from build123d import *

# Parameters (mm, degrees)
CYLINDER040_R     = 3.25
CYLINDER040_DEPTH = 2
CYLINDER041_R     = 3.25
CYLINDER041_DEPTH = 2
CYLINDER042_R     = 3.25
CYLINDER042_DEPTH = 2
CYLINDER039_R     = 3.25
CYLINDER039_DEPTH = 2
CYLINDER035_R     = 1.27
CYLINDER035_DEPTH = 5
CYLINDER037_R     = 1.27
CYLINDER037_DEPTH = 5
CYLINDER038_R     = 1.27
CYLINDER038_DEPTH = 5
CYLINDER036_R     = 1.27
CYLINDER036_DEPTH = 5
BOX021_W          = 7
BOX021_H          = 8
BOX021_DEPTH      = 2
BOX022_W          = 7
BOX022_H          = 8
BOX022_DEPTH      = 2
BOX020_W          = 7
BOX020_H          = 23
BOX020_DEPTH      = 2
BOX019_W          = 40
BOX019_H          = 25
BOX019_DEPTH      = 3


with BuildPart() as cylinder040:
    # Cylinder040 → Cylinder040 (new body)
    with BuildSketch(Plane(origin=(3.54, 3.54, 0), x_dir=(1, 0, 0), z_dir=(0, 0, 1))):
        Circle(CYLINDER040_R)
    extrude(amount=CYLINDER040_DEPTH)


with BuildPart() as cylinder041:
    # Cylinder041 → Cylinder041 (new body)
    with BuildSketch(Plane(origin=(34.7, 18.5, 0), x_dir=(1, 0, 0), z_dir=(0, 0, 1))):
        Circle(CYLINDER041_R)
    extrude(amount=CYLINDER041_DEPTH)


with BuildPart() as cylinder042:
    # Cylinder042 → Cylinder042 (new body)
    with BuildSketch(Plane(origin=(34.7, 5.06, 0), x_dir=(1, 0, 0), z_dir=(0, 0, 1))):
        Circle(CYLINDER042_R)
    extrude(amount=CYLINDER042_DEPTH)


with BuildPart() as washer_bolt_holes:
    # Cylinder039 → Cylinder039 (new body)
    with BuildSketch(Plane(origin=(3.54, 20.05, 0), x_dir=(1, 0, 0), z_dir=(0, 0, 1))):
        Circle(CYLINDER039_R)
    extrude(amount=CYLINDER039_DEPTH)

    # Fusion023: union Cylinder040, Cylinder041, Cylinder042
    add(cylinder040.part)
    add(cylinder041.part)
    add(cylinder042.part)


with BuildPart() as cylinder035:
    # Cylinder035 → Cylinder035 (new body)
    with BuildSketch(Plane(origin=(2.54, 19.05, 0), x_dir=(1, 0, 0), z_dir=(0, 0, 1))):
        Circle(CYLINDER035_R)
    extrude(amount=CYLINDER035_DEPTH)


with BuildPart() as cylinder037:
    # Cylinder037 → Cylinder037 (new body)
    with BuildSketch(Plane(origin=(33.7, 17.5, 0), x_dir=(1, 0, 0), z_dir=(0, 0, 1))):
        Circle(CYLINDER037_R)
    extrude(amount=CYLINDER037_DEPTH)


with BuildPart() as cylinder038:
    # Cylinder038 → Cylinder038 (new body)
    with BuildSketch(Plane(origin=(33.7, 4.064, 0), x_dir=(1, 0, 0), z_dir=(0, 0, 1))):
        Circle(CYLINDER038_R)
    extrude(amount=CYLINDER038_DEPTH)


with BuildPart() as complete_blackplate_holes:
    # Cylinder036 → Cylinder036 (new body)
    with BuildSketch(Plane(origin=(2.54, 2.54, 0), x_dir=(1, 0, 0), z_dir=(0, 0, 1))):
        Circle(CYLINDER036_R)
    extrude(amount=CYLINDER036_DEPTH)

    # Fusion021: union Cylinder035, Cylinder037, Cylinder038
    add(cylinder035.part)
    add(cylinder037.part)
    add(cylinder038.part)


with BuildPart() as complete_blackplate_holes_1:
    # Fusion021 placement: moved
    add(complete_blackplate_holes.part.moved(Location((1, 1, 0))))

    # Fusion024: union Washer Bolt Holes
    add(washer_bolt_holes.part)


with BuildPart() as cube012:
    # Box021 → Box021 (new body)
    with BuildSketch(Plane(origin=(31, 15, 3), x_dir=(1, 0, 0), z_dir=(0, 0, 1))):
        with Locations((3.5, 4)):
            Rectangle(BOX021_W, BOX021_H)
    extrude(amount=BOX021_DEPTH)


with BuildPart() as cube013:
    # Box022 → Box022 (new body)
    with BuildSketch(Plane(origin=(31, 0, 3), x_dir=(1, 0, 0), z_dir=(0, 0, 1))):
        with Locations((3.5, 4)):
            Rectangle(BOX022_W, BOX022_H)
    extrude(amount=BOX022_DEPTH)


with BuildPart() as standoff_blocks:
    # Box020 → Box020 (new body)
    with BuildSketch(Plane.XY.offset(3)):
        with Locations((3.5, 11.5)):
            Rectangle(BOX020_W, BOX020_H)
    extrude(amount=BOX020_DEPTH)

    # Fusion022: union Cube012, Cube013
    add(cube012.part)
    add(cube013.part)


with BuildPart() as regulator_base:
    # Box019 → Box019 (new body)
    with BuildSketch(Plane(origin=(-1, -1, 0), x_dir=(1, 0, 0), z_dir=(0, 0, 1))):
        with Locations((20, 12.5)):
            Rectangle(BOX019_W, BOX019_H)
    extrude(amount=BOX019_DEPTH)

    # Fusion025: union Standoff Blocks
    add(standoff_blocks.part)

    # Cut012: cut Complete Blackplate Holes
    add(complete_blackplate_holes_1.part, mode=Mode.SUBTRACT)


with BuildPart() as regulator_base_1:
    # Cut012 placement: moved
    add(regulator_base.part.moved(Location((12.5, 63, 3))))


solid = regulator_base_1.part
Can you work these out from the model? Positions are in its coordinate system, mm. A direction names the side the tool comes from. Give positions to 0.01 mm unless a question says otherwise; leave off trailing zeros. Loops run counter-clockwise (first coordinate to the right, second up) from the corner with the lowest first, then second, coordinate; pieces in that order, holes last. Notation, with made-up numbers: (-23.5, 62.5) - (3.5, 62.5) arc R25 ccw to (3.5, 97.5) - close; hole circle Ø9 at (7.25, -19.5). An arc over 180 degrees is marked (long way). Return JSON: item names as keys, results as strings.
1. I want a section at A-A on x = 47.2. Please give me the cut outline in (y, z), and give its area (3 significant figures).
Output values:
{"outline": "(62, 3) - (64.81, 3) - (64.81, 5) - (66.79, 5) - (66.79, 8) - (63, 8) - (63, 6) - (62, 6) - close; (69.33, 5) - (71.31, 5) - (71.31, 3) - (78.25, 3) - (78.25, 5) - (80.23, 5) - (80.23, 8) - (78, 8) - (78, 6) - (71, 6) - (71, 8) - (69.33, 8) - close; (82.77, 5) - (84.75, 5) - (84.75, 3) - (87, 3) - (87, 6) - (86, 6) - (86, 8) - (82.77, 8) - close", "area": "65.8 mm²"}
2. We'd pull the mould along X, two halves only. Please class faces 1 (the face through (11.5, 74, 4)), 2 (the face through (50.5, 82, 7)), 3 (the face through (43.5, 67, 7)), 4 (the face through (47, 78, 7)): +X half, -X half, draft (parallel to the pull), parting line (faces both ways), or undercut.
Output values:
{"face 1": "-X half", "face 2": "+X half", "face 3": "undercut", "face 4": "draft"}
3. For faces 5 (the face through (47, 63, 7)), 6 (the face through (19.5, 74, 7)), 7 (the face through (17, 82, 5)), which set-ups out of +Z, -Z, +X, -X, +Y, -Y let a thin tool reach every point of the face, with its end or its side?
Output values:
{"face 5": "+Z, +X, -X, -Y", "face 6": "+Z, +Y, -Y", "face 7": "-Z"}
4. If I drill on line 1 (Y direction, x = 16.04, z = 4.5); line 2 (Y direction, x = 47.2, z = 4.2); line 3 (X direction, y = 66.54, z = 7), over which ranges is the centre line in solid material (lowest first)?
Output values:
{"line 1": "y = 62 to 63.29, 69.79 to 79.8, 86.3 to 87", "line 2": "y = 62 to 64.81, 71.31 to 78.25, 84.75 to 87", "line 3": "x = 12.5 to 14.77, 17.31 to 19.5, 43.5 to 50.5"}
5. I want a section at C-C on z = 3.75. Please give me the cut outline in (x, y), and give its area (3 significant figures).
Output values:
{"outline": "(11.5, 62) - (51.5, 62) - (51.5, 87) - (11.5, 87) - close; hole circle Ø6.5 at (16.04, 66.54); hole circle Ø6.5 at (16.04, 83.05); hole circle Ø6.5 at (47.2, 68.06); hole circle Ø6.5 at (47.2, 81.5)", "area": "867 mm²"}
6. I'm going to push flat-ended pins straight in: pin 1 Ø4 at (x, y) = (16.04, 83.05) entering from +Z; pin 2 Ø0.6 at (x, z) = (15, 7.5) entering from +Y; pin 3 Ø1.6 at (x, z) = (47.5, 7) entering from -Y; pin 4 Ø3 at (x, y) = (47.2, 81.5) entering from -Z. Where does each tip first touch, or does it pass through?
Output values:
{"pin 1": "stops at z = 8", "pin 2": "stops at y = 86", "pin 3": "stops at y = 63", "pin 4": "stops at z = 5"}
7. I want a section at D-D on y = 77. Please give me the cut outline in (x, z).
Output values:
{"outline": "(11.5, 3) - (51.5, 3) - (51.5, 6) - (19.5, 6) - (19.5, 8) - (12.5, 8) - (12.5, 6) - (11.5, 6) - close"}
8. I want a section at B-B on z = 7.6. Please give me the cut outline in (x, y), and give its area (3 significant figures).
Output values:
{"outline": "(12.5, 63) - (19.5, 63) - (19.5, 86) - (12.5, 86) - close; (43.5, 63) - (50.5, 63) - (50.5, 71) - (43.5, 71) - close; (43.5, 78) - (50.5, 78) - (50.5, 86) - (43.5, 86) - close; hole circle Ø2.54 at (16.04, 66.54); hole circle Ø2.54 at (16.04, 83.05); hole circle Ø2.54 at (47.2, 68.06); hole circle Ø2.54 at (47.2, 81.5)", "area": "253 mm²"}
